The drawing under review shows one solid part. Ordinate dimensions are in mm from its lowest x, y, z. A direction names the side the tool comes from. Give positions to 0.01 mm unless a question says otherwise; leave off trailing zeros. Write each loop counter-clockwise with the first axis right and the second up, starting at its lowest first coordinate (ties: lowest second). Pieces come first, ordered by that corner, then holes. Notation, with made-up numbers: M 1.5,-25.5 L 24.5,-25.5 A22 ccw 24.5,-1.5 Z; hole C -27.75,64.5 d9. An arc over 180 degrees is marked long. Write item = value, one per line. Start each with the question number.
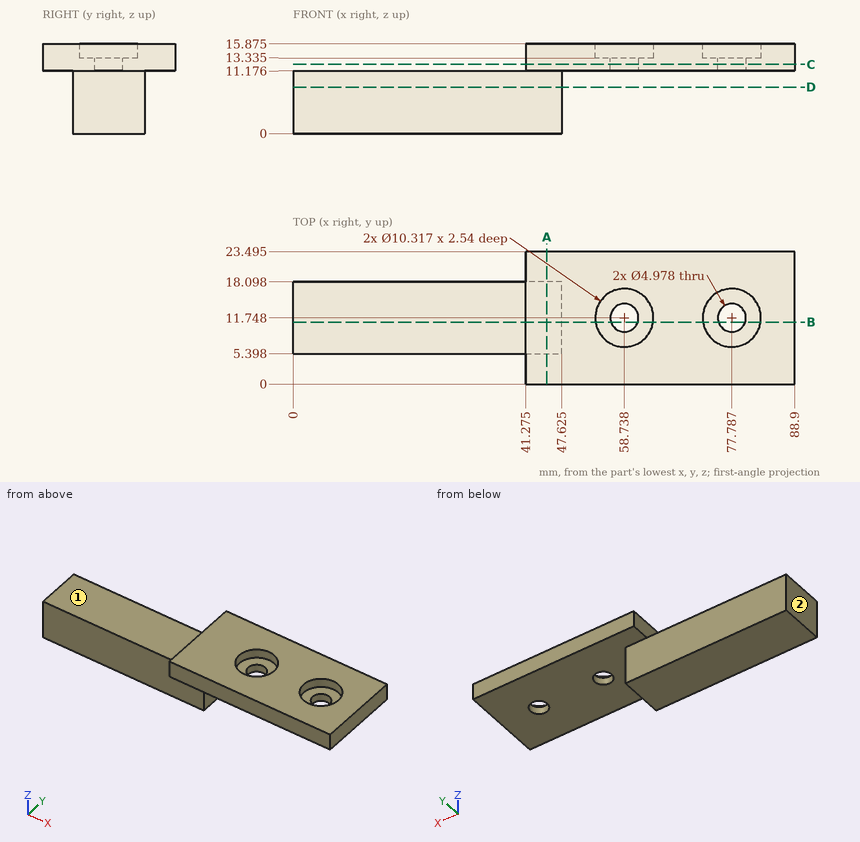
Item 1: We need section C-C, the plane z = 12.25. Write out the cut boundary in (x, y) (1 decimal), and give its area (3 significant figures).
Item 2: We need section D-D, the plane z = 8.25. Write out the cut boundary in (x, y) (1 decimal).
Item 3: We need section B-B, the plane y = 11. Write out the cut boundary in (x, z) (1 decimal).
Item 4: We need section A-A, the plane x = 45. Write out the cut boundary in (y, z) (1 decimal).
Item 5: To check wall thickness, follow probe 1 along X at (y, z) = (11, 11.5) (1 decimal); probe 2 along Z at (x, y) = (15, 11.5) (1 decimal); probe 3 along Y at (x, z) = (33.5, 10.25). State the ranges of each line that lie inside material, in increasing order. Write a range as [from, to].
Item 6: Clearance check with flat-ended pins moving along their axes: P1, Ø5, axis at x = 57.5, y = 13.5, coming from the +Z side (1 decimal); P2, Ø5.5, axis at x = 77.79, y = 11.75, coming from the -Z side; P3, Ø2, axis at y = 5.5, z = 9, coming from the +X side (1 decimal); P4, Ø4, axis at x = 58.74, y = 11.75, coming from the -Z side. State where each tip first meets the part, or that it passes through.
Item 7: For the marked faces 1 and 2, list the 3-axis set-ups (+Z, -Z, +X, -X, +Y, -Y) from which the entire face can be reached by the end or side of a thin tool; tool diameter is ignored.
Worked out:
q1.outline = M 41.3,0 L 88.9,0 L 88.9,23.5 L 41.3,23.5 Z; hole C 58.7,11.7 d5; hole C 77.8,11.7 d5
q1.area = 1,080 mm²
q2.outline = M 0,5.4 L 47.6,5.4 L 47.6,18.1 L 0,18.1 Z
q3.outline = M 0,0 L 47.6,0 L 47.6,11.2 L 56.4,11.2 L 56.4,13.3 L 53.6,13.3 L 53.6,15.9 L 41.3,15.9 L 41.3,11.2 L 0,11.2 Z; M 61.1,11.2 L 75.4,11.2 L 75.4,13.3 L 72.7,13.3 L 72.7,15.9 L 63.8,15.9 L 63.8,13.3 L 61.1,13.3 Z; M 80.2,11.2 L 88.9,11.2 L 88.9,15.9 L 82.9,15.9 L 82.9,13.3 L 80.2,13.3 Z
q4.outline = M 0,11.2 L 5.4,11.2 L 5.4,0 L 18.1,0 L 18.1,11.2 L 23.5,11.2 L 23.5,15.9 L 0,15.9 Z
q5.probe_1 = [41.3, 56.4], [61.1, 75.4], [80.2, 88.9]
q5.probe_2 = [0, 11.2]
q5.probe_3 = [5.4, 18.1]
q6.P1 = 13.3
q6.P2 = 11.18
q6.P3 = 47.6
q6.P4 = through
q7.face_1 = +Z, -X, +Y, -Y
q7.face_2 = +Z, -Z, -X, +Y, -Y
